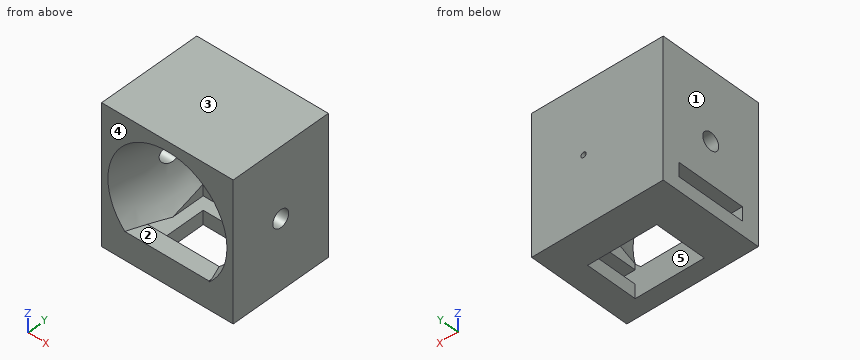
Autodesk Inventor part; units mm, degrees
ref_plane "YZ Plane" through (0, 0, 0) normal (1, 0, 0) x (0, 1, 0)
ref_plane "XZ Plane" through (0, 0, 0) normal (0, 1, 0) x (-1, 0, 0)
ref_plane "XY Plane" through (0, 0, 0) normal (0, 0, 1) x (1, 0, 0)
ref_plane "Work Plane13" through (0, 3, 0) normal (0, 1, 0) x (1, 0, 0)
sketch "Sketch45" plane through (0, 3, 0) normal (0, 1, 0) x (1, 0, 0)
  line L0 (35, -20) -> (-3, -20)
  line L1 (-3, -20) -> (-3, 20)
  line L2 (-3, 20) -> (35, 20)
  line L3 (35, 20) -> (35, -20)
  point P0 (0, 0)
  dimension "d142" = 38
  dimension "d143" = 40
extrude "Extrusion34" add sketch "Sketch45" along normal blind 30
sketch "Sketch46" plane through (0, 33, 0) normal (0, 1, 0) x (1, 0, 0)
  point P0 (0, 0)
ref_plane "Work Plane11" through (0, 0, 0) normal (0, -1, 0) x (1, 0, 0)
sketch "Sketch47" plane through (0, 0, 0) normal (0, -1, 0) x (1, 0, 0)
  circle A0 centre (16, 0) radius 18
  point P0 (0, 0)
  dimension "d146" = 36
extrude "Extrusion35" cut sketch "Sketch47" against normal blind 30 draft -15
sketch "Sketch48" plane through (0, 33, 0) normal (0, 1, 0) x (1, 0, 0)
  point P0 (0, 0)
sketch "Sketch49" plane through (0, 33, 0) normal (0, 1, 0) x (1, 0, 0)
  circle A0 centre (20, 0) radius 0.75
  point P0 (0, 0)
  dimension "d149" = 1.5
extrude "Extrusion36" cut sketch "Sketch49" against normal through all
ref_plane "Work Plane7" through (35, 3, -20) normal (0, 0, -1) x (-1, 0, 0)
sketch "Sketch58" plane through (35, 3, -20) normal (0, 0, -1) x (-1, 0, 0)
  line L0 (7, 20) -> (27, 20)
  line L1 (27, 20) -> (27, 5)
  line L2 (27, 5) -> (7, 5)
  line L3 (7, 5) -> (7, 20)
  point P0 (35, -3)
  dimension "d156" = 20
  dimension "d157" = 15
extrude "Extrusion38" cut sketch "Sketch58" against normal blind 15
ref_plane "Work Plane4" through (-3, 3, -20) normal (-1, 0, 0) x (0, 0, 1)
sketch "Sketch59" plane through (-3, 3, -20) normal (-1, 0, 0) x (0, 0, 1)
  line L0 (4, 25) -> (8, 25)
  line L1 (8, 25) -> (8, 5)
  line L2 (8, 5) -> (4, 5)
  line L3 (4, 5) -> (4, 25)
  point P0 (20, -3)
  dimension "d160" = 4
  dimension "d161" = 20
extrude "Extrusion39" cut sketch "Sketch59" against normal blind 35
ref_plane "Work Plane1" through (0, 3, 0) normal (0, 1, 0) x (1, 0, 0)
ref_plane "Work Plane6" through (0, 23, 0) normal (0, 1, 0) x (1, 0, 0)
sketch "Sketch62" plane through (-3, 3, -20) normal (-1, 0, 0) x (0, 0, 1)
  circle A0 centre (20, 15) radius 2.5
  point P0 (20, -3)
  dimension "d172" = 5
extrude "Extrusion42" cut sketch "Sketch62" against normal through all
sketch "Sketch65" plane through (0, 3, 0) normal (0, -1, 0) x (1, 0, 0)
  line L0 (-3, -12) -> (32, -12)
  line L1 (28, -20) -> (28, -16)
  line L2 (3.5815, -12) -> (28, -12)
  line L3 (28, -12) -> (28, -17.2375)
  line L4 (28, -17.2375) -> (3.5815, -17.2375)
  line L5 (3.5815, -17.2375) -> (3.5815, -12)
  point P0 (0, 0)
extrude "Extrusion44" add sketch "Sketch65" against normal blind 5
properties part number "liquid port_only_v03"
Part model, mm, in its own coordinate system. Face numbers are marked on the shaded views. A direction names the side the tool comes from. Coordinates: 2 decimals unless noted, no trailing zeros. Order: outer loops, then holes, each group sorted by start corner. A loop starts at its lowest first (then second) coordinate and runs counter-clockwise, first axis right, second up.
(1) Tool access for the marked faces 1 and 2: list every direction of +Z, -Z, +X, -X, +Y, -Y with a clear straight run to the whole face (end or side of a thin tool).
Check sheet entries:
face 1: +Z, -Z, -X, +Y, -Y
face 2: -Y
(2) Slice it at C-C, the plane x = 16. Write the cut outline in (y, z).
Check sheet entries:
outline: (3, -20) - (8, -20) - (8, -12) - (3, -12) - close; (3, 17.2) - (30, 9.96) - (30, -9.96) - (23, -11.84) - (23, -12) - (28, -12) - (28, -16) - (23, -16) - (23, -20) - (33, -20) - (33, 20) - (3, 20) - close
(3) Slice it at A-A, the plane y = 18. Write the cut outline in (x, z), and give its area (3 significant figures).
Check sheet entries:
outline: (-3, -20) - (8, -20) - (8, -16) - (-3, -16) - close; (-3, -12) - (8, -12) - (8, -10.47) arc R13.18 cw to (3.06, -2.5) - (-3, -2.5) - close; (-3, 2.5) - (3.06, 2.5) arc R13.18 cw to (28.94, 2.5) - (35, 2.5) - (35, 20) - (-3, 20) - close; (28, -20) - (35, -20) - (35, -2.5) - (28.94, -2.5) arc R13.18 cw to (28, -5.44) - (28, -12) - (32, -12) - (32, -16) - (28, -16) - close
area: 686 mm2
(4) Slice it at D-D, the plane x = 20. State how many separate pieces and enclosed holes the cut face has, and give its area (3 significant figures).
Check sheet entries:
separate pieces: 3
enclosed holes: 0
area: 395 mm2
(5) Pin check, flat tips, straight feed: pin 1 Ø1.5 at (x, y) = (14, 22.5) entering from -Z; pin 2 Ø1.4 at (x, y) = (27, 21) entering from -Z; pin 3 Ø3 at (y, z) = (18, 0) entering from +X. Stop position of each tip, or through.
Check sheet entries:
pin 1: stops at z = -20
pin 2: stops at z = -5
pin 3: passes through
(6) Probe L1, parallel to Z at x = -0.5, y = 18; L2, parallel to Z at x = 20, y = 30.9; L3, parallel to Z at x = 2.5, y = 24. List the from-to ranges inside material, lowest first.
Check sheet entries:
L1: z = -20 to -16, -12 to -2.5, 2.5 to 20
L2: z = -20 to -0.75, 0.75 to 20
L3: z = -20 to -16, -12 to 20
(7) Pull direction Y, two halves, no side cores. Call the marked faces 3, 4 and 5: pulls with the +Y half, pulls with the -Y half, needs draft (parallel to the pull), parting line crosses it, or undercut.
Check sheet entries:
face 3: needs draft
face 4: pulls with the -Y half
face 5: undercut
(8) Slice it at B-B, the plane z = 0. Write the cut outline in (x, y).
Check sheet entries:
outline: (-3, 3) - (-1.2, 3) - (2.15, 15.5) - (-3, 15.5) - close; (-3, 20.5) - (3.49, 20.5) - (6.04, 30) - (19.25, 30) - (19.25, 33) - (-3, 33) - close; (20.75, 30) - (25.96, 30) - (28.51, 20.5) - (35, 20.5) - (35, 33) - (20.75, 33) - close; (29.85, 15.5) - (33.2, 3) - (35, 3) - (35, 15.5) - close
